For this review, take the finished solid that the model builds, in its own axes (mm). Give positions to 0.01 mm unless a question says otherwise; leave off trailing zeros. Order: outer loops, then holes, each group sorted by start corner. A loop starts at its lowest first (then second) coordinate and runs counter-clockwise, first axis right, second up. Notation, with made-up numbers: (-29.5, 43.5) -> (12.5, 43.5) arc R23 ccw to (12.5, 51.5) -> close; hole circle Ø4 at (-23, 30). An arc over 180 degrees is marked (long way). Return JSON: item names as keys, results as strings. Group by question number.
1) Add section B-B (z = 4). Give the boundary of the cut face in (x, y).
2) Add section C-C (y = 4.6). State how many separate pieces and enclosed holes the cut face has, then the cut area to 3 significant figures.
3) Insertion check: P1, Ø5, axis at x = 43.5, z = -8, coming from the -Y side. The pin has a flat end and moves straight along its axis. Give the tip position at first contact, or say it passes through.
4) Add section A-A (x = 0). Give the boundary of the cut face in (y, z), then the cut area to 3 significant figures.
5) To check wall thickness, follow line 1 along X through (y, z) = (1.8, -15); line 2 along Z through (x, y) = (0, 3.95); line 3 along X through (y, z) = (2.15, 5.5). State the ranges of each line that lie inside material, in increasing order.
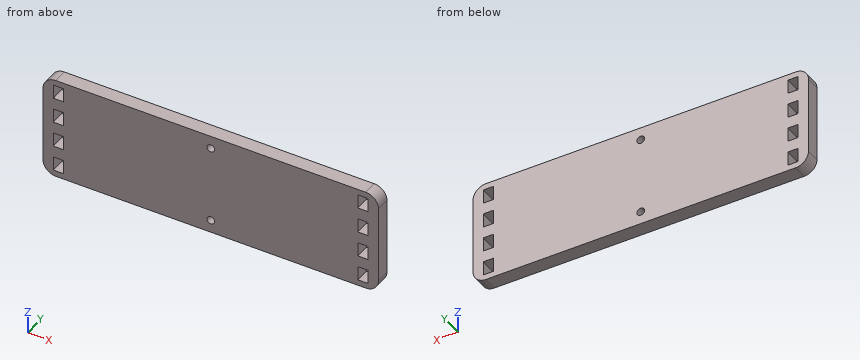
from build123d import *

# Parameters (mm, degrees)
SKETCH1_W           = 130
SKETCH1_H           = 40
SKETCH1_R           = 1.5
BOSS_EXTRUDE1_DEPTH = 5.5
SKETCH2_W           = 4
SKETCH2_H           = 5.5
CUT_EXTRUDE1_DEPTH  = 6.5
FILLET1_R           = 5


with BuildPart() as part:
    # Sketch1 → Boss-Extrude1 (new body)
    with BuildSketch(Plane(origin=(0, 0, 0), x_dir=(1, 0, 0), z_dir=(0, 1, 0))):
        Rectangle(SKETCH1_W, SKETCH1_H)
        with Locations((0, 15)):
            Circle(SKETCH1_R, mode=Mode.SUBTRACT)
        with Locations((0, -15)):
            Circle(SKETCH1_R, mode=Mode.SUBTRACT)
    extrude(amount=BOSS_EXTRUDE1_DEPTH)

    # Sketch2 → Cut-Extrude1 (cut, through all)
    with BuildSketch(Plane(origin=(0, 5.5, 0), x_dir=(1, 0, 0), z_dir=(0, 1, 0))):
        with Locations((-59, 5)):
            Rectangle(SKETCH2_W, SKETCH2_H)
        with Locations((-59, 15)):
            Rectangle(SKETCH2_W, SKETCH2_H)
        with Locations((-59, -5)):
            Rectangle(SKETCH2_W, SKETCH2_H)
        with Locations((-59, -15)):
            Rectangle(SKETCH2_W, SKETCH2_H)
        with Locations((59, -15)):
            Rectangle(SKETCH2_W, SKETCH2_H)
        with Locations((59, 15)):
            Rectangle(SKETCH2_W, SKETCH2_H)
        with Locations((59, -5)):
            Rectangle(SKETCH2_W, SKETCH2_H)
        with Locations((59, 5)):
            Rectangle(SKETCH2_W, SKETCH2_H)
    extrude(amount=-CUT_EXTRUDE1_DEPTH, mode=Mode.SUBTRACT)

    # Fillet1
    fillet1_edges = [part.edges().sort_by_distance(p)[0] for p in [
        (-65, 2.75, -20),
        (65, 2.75, -20),
        (65, 2.75, 20),
        (-65, 2.75, 20),
    ]]
    fillet(fillet1_edges, radius=FILLET1_R)


solid = part.part
Evaluation:
{
 "1": {"outline": "(-65, 0) -> (-61, 0) -> (-61, 5.5) -> (-65, 5.5) -> close; (-57, 0) -> (57, 0) -> (57, 5.5) -> (-57, 5.5) -> close; (61, 0) -> (65, 0) -> (65, 5.5) -> (61, 5.5) -> close"},
 "2": {"separate pieces": "1", "enclosed holes": "10", "area": "4,990 mm^2"},
 "3": {"P1": "y = 0"},
 "4": {"outline": "(0, -20) -> (5.5, -20) -> (5.5, -16.5) -> (0, -16.5) -> close; (0, -13.5) -> (5.5, -13.5) -> (5.5, 13.5) -> (0, 13.5) -> close; (0, 16.5) -> (5.5, 16.5) -> (5.5, 20) -> (0, 20) -> close", "area": "187 mm^2"},
 "5": {"line 1": "-65 to -61, -57 to -1.5, 1.5 to 57, 61 to 65", "line 2": "-20 to -16.5, -13.5 to 13.5, 16.5 to 20", "line 3": "-65 to -61, -57 to 57, 61 to 65"}
}
